Design review of the part shown in the three views and the two pictorial views. Dimensions are in mm from the part's minimum x, y and z. A direction names the side the tool comes from. Round coordinates to 2 decimals unless told otherwise and drop trailing zeros. Order: outer loops, then holes, each group sorted by start corner. A loop starts at its lowest first (then second) coordinate and runs counter-clockwise, first axis right, second up.
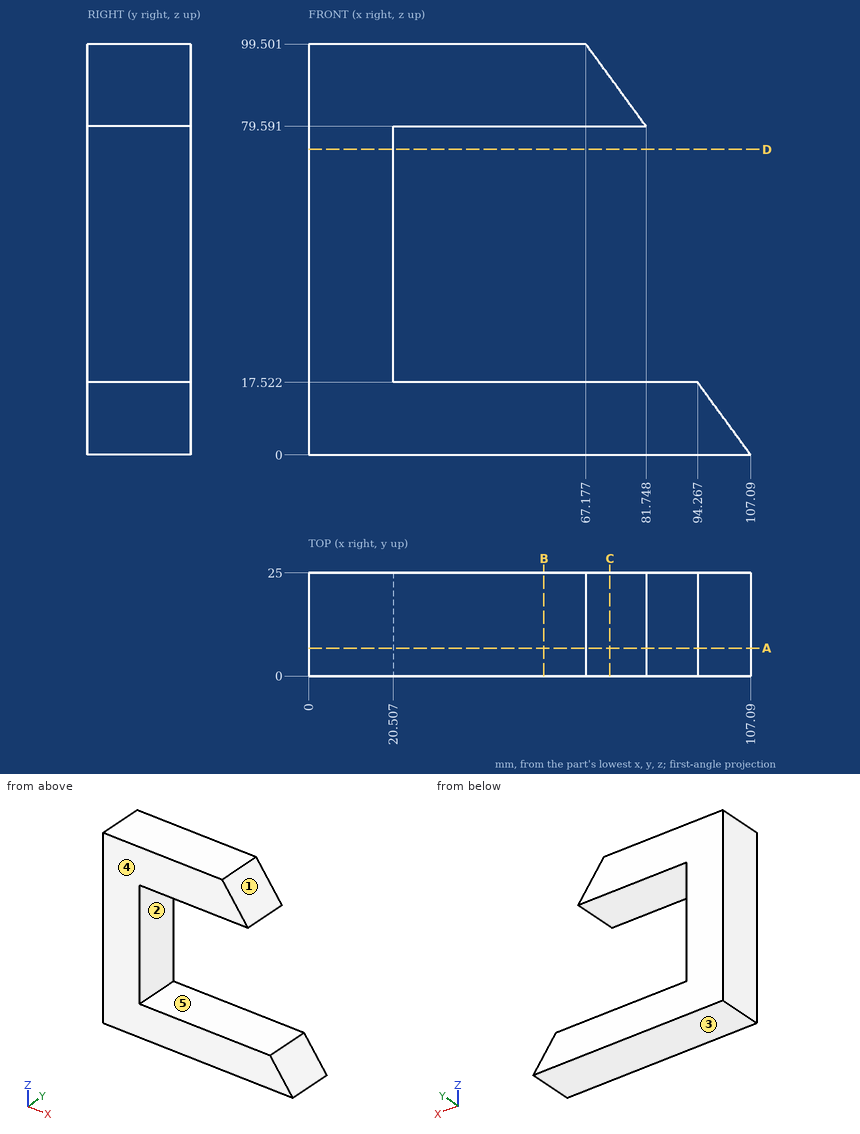
(1) Insertion check: pin 1 (3 mm diameter, centred on x = 84, y = 13.5, fed in from +Z). The pin has a flat end and moves straight along its axis. Give the tip position at first contact, or say it passes through.
Data:
pin 1: stops at z = 17.52
(2) To check wall thickness, follow probe 1 along Z at (x, y) = (55, 12.5); probe 2 along Z at (x, y) = (71, 1.5) (1 decimal); probe 3 along X at (y, z) = (5.25, 51.5). State the ranges of each line that lie inside material, in increasing order.
Data:
probe 1: z = 0 to 17.52, 79.59 to 99.5
probe 2: z = 0 to 17.5, 79.6 to 94.3
probe 3: x = 0 to 20.51
(3) Consider section B-B (x = 57). Write out the cut boundary in (y, z).
Data:
outline: (0, 0) - (25, 0) - (25, 17.52) - (0, 17.52) - close; (0, 79.59) - (25, 79.59) - (25, 99.5) - (0, 99.5) - close
(4) Consider section D-D (z = 74). Write out the cut boundary in (x, y).
Data:
outline: (0, 0) - (20.51, 0) - (20.51, 25) - (0, 25) - close
(5) Consider section C-C (x = 73). Write out the cut boundary in (y, z), and give its area (3 significant figures).
Data:
outline: (0, 0) - (25, 0) - (25, 17.52) - (0, 17.52) - close; (0, 79.59) - (25, 79.59) - (25, 91.54) - (0, 91.54) - close
area: 737 mm2
(6) For the marked faces 4 and 5, list the 3-axis set-ups (+Z, -Z, +X, -X, +Y, -Y) from which the entire face can be reached by the end or side of a thin tool; tool diameter is ignored.
Data:
face 4: +Z, -Z, +X, -X, -Y
face 5: +X, +Y, -Y
(7) Draft analysis for pull direction Z (two halves, no side actions). For the marked faces 1, 2 and 3, state which applies: pulls with the +Z half, pulls with the -Z half, needs draft (parallel to the pull), parting line crosses it, or undercut.
Data:
face 1: pulls with the +Z half
face 2: undercut
face 3: pulls with the -Z half
(8) Consider section A-A (y = 6.75). Write out the cut boundary in (x, z), and give its area (3 significant figures).
Data:
outline: (0, 0) - (107.09, 0) - (94.27, 17.52) - (20.51, 17.52) - (20.51, 79.59) - (81.75, 79.59) - (67.18, 99.5) - (0, 99.5) - close
area: 4,520 mm2
